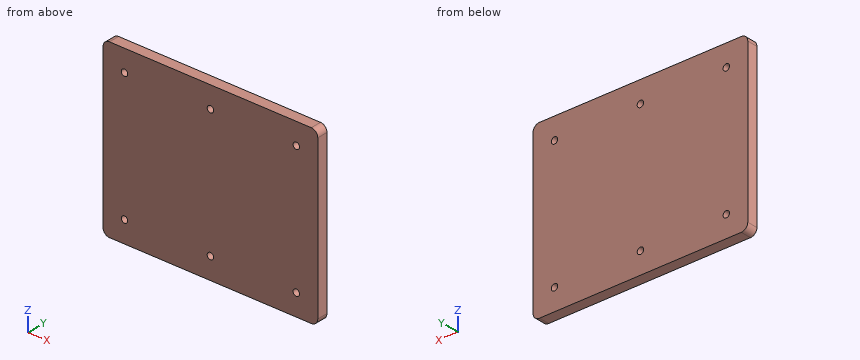
from build123d import *

# Parameters (mm, degrees)
SKETCH_2_W      = 100
SKETCH_2_H      = 80
SKETCH_2_R      = 1.5
EXTRUDE_1_DEPTH = 5
FILLET_1_R      = 3


with BuildPart() as part:
    # 草图2 → 凸台-拉伸1 (new body)
    with BuildSketch(Plane(origin=(0, 0, 0), x_dir=(1, 0, 0), z_dir=(0, 1, 0))):
        with Locations((50, 40)):
            Rectangle(SKETCH_2_W, SKETCH_2_H)
        with Locations((10, 10)):
            Circle(SKETCH_2_R, mode=Mode.SUBTRACT)
        with Locations((50, 10)):
            Circle(SKETCH_2_R, mode=Mode.SUBTRACT)
        with Locations((90, 10)):
            Circle(SKETCH_2_R, mode=Mode.SUBTRACT)
        with Locations((90, 70)):
            Circle(SKETCH_2_R, mode=Mode.SUBTRACT)
        with Locations((50, 70)):
            Circle(SKETCH_2_R, mode=Mode.SUBTRACT)
        with Locations((10, 70)):
            Circle(SKETCH_2_R, mode=Mode.SUBTRACT)
    extrude(amount=EXTRUDE_1_DEPTH)

    # 圆角1
    fillet_1_edges = [part.edges().sort_by_distance(p)[0] for p in [
        (0, 2.5, -80),
        (100, 2.5, -80),
        (100, 2.5, 0),
        (0, 2.5, 0),
    ]]
    fillet(fillet_1_edges, radius=FILLET_1_R)


solid = part.part
Geometry check sheet. Reference: the model listing, model coordinates, mm. Round coordinates to 2 decimals unless told otherwise and drop trailing zeros. Loops run counter-clockwise (first coordinate to the right, second up) from the corner with the lowest first, then second, coordinate; pieces in that order, holes last.
Item 1: Cross-section at A-A on z = -10. Record the boundary of the cut face in (x, y).
Item 2: Gauge pin test, flat end, axial feed: pin 1 (1.8 mm diameter, centred on x = 10, z = -70, fed in from +Y). Record the tip position at first contact, or that the pin passes through.
Item 3: Thickness scan on line 1 (X direction, y = 1.35, z = -70); line 2 (Z direction, x = 90, y = 3.95); line 3 (Z direction, x = 9.5, y = 0.2). Record the ranges inside material, lowest first.
Item 4: Cross-section at B-B on x = 10. Record the boundary of the cut face in (y, z).
Answer sheet:
1. outline: (0, 0) - (8.5, 0) - (8.5, 5) - (0, 5) - close; (11.5, 0) - (48.5, 0) - (48.5, 5) - (11.5, 5) - close; (51.5, 0) - (88.5, 0) - (88.5, 5) - (51.5, 5) - close; (91.5, 0) - (100, 0) - (100, 5) - (91.5, 5) - close
2. pin 1: passes through
3. line 1: x = 0 to 8.5, 11.5 to 48.5, 51.5 to 88.5, 91.5 to 100
3. line 2: z = -80 to -71.5, -68.5 to -11.5, -8.5 to 0
3. line 3: z = -80 to -71.41, -68.59 to -11.41, -8.59 to 0
4. outline: (0, -80) - (5, -80) - (5, -71.5) - (0, -71.5) - close; (0, -68.5) - (5, -68.5) - (5, -11.5) - (0, -11.5) - close; (0, -8.5) - (5, -8.5) - (5, 0) - (0, 0) - close
